Geometry check sheet. Reference: drawing and pictorial views, mm from the part's lowest x, y, z. Coordinates: 2 decimals unless noted, no trailing zeros. Loops run counter-clockwise (first coordinate to the right, second up) from the corner with the lowest first, then second, coordinate; pieces in that order, holes last. Notation, with made-up numbers: (-22, 89) - (1, 89) arc R24 ccw to (1, 100) - close; hole circle Ø7 at (14.25, 34.25). An arc over 180 degrees is marked (long way). One line per item, written item: value.
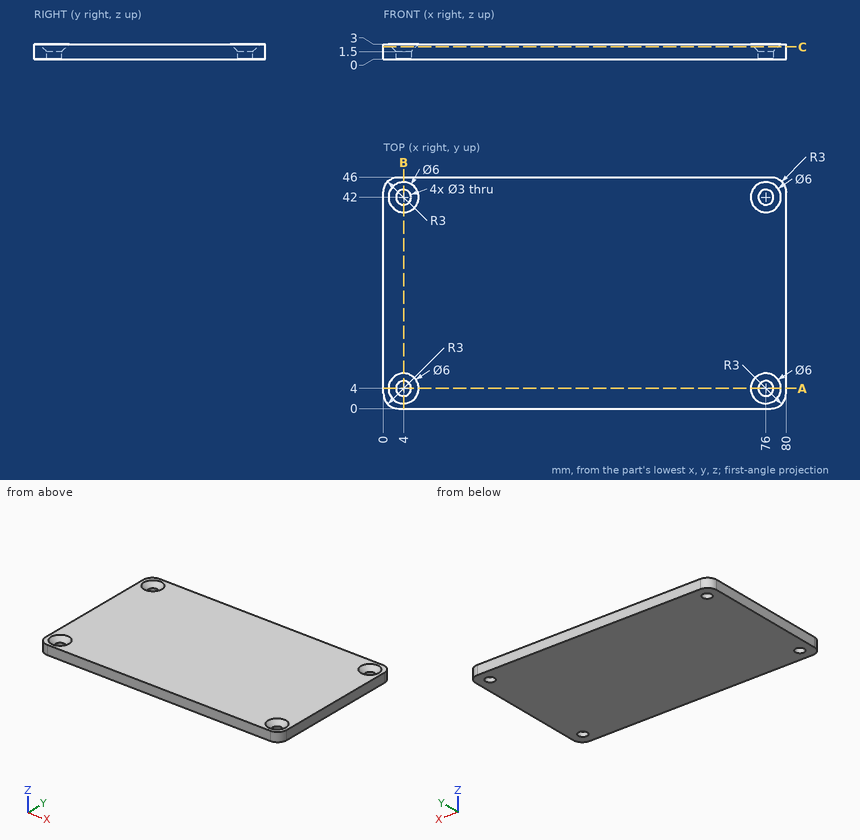
(1) Material ranges on probe 1 along Y at (x, z) = (4, 1.15); probe 2 along Y at (x, z) = (75.5, 2.1); probe 3 along X at (y, z) = (43.5, 2.4), recorded low to high. Write a range as from..to.
Reply:
probe 1: 0..2.5, 5.5..40.5, 43.5..46
probe 2: 0..1.96, 6.04..39.96, 44.04..46
probe 3: 0.04..2.13, 5.87..74.13, 77.87..79.96
(2) Go/stop test with flat-tipped pins: pin 1 Ø2.5 at (x, y) = (4, 42) entering from -Z; pin 2 Ø5 at (x, y) = (4, 4) entering from -Z. Record where each tip stops, or that it passes through.
Reply:
pin 1: through
pin 2: z = 0
(3) Cross-section at B-B on x = 4. Record the cut outline in (y, z).
Reply:
outline: (0, 0) - (2.5, 0) - (2.5, 1.5) - (1, 3) - (0, 3) - close; (5.5, 0) - (40.5, 0) - (40.5, 1.5) - (39, 3) - (7, 3) - (5.5, 1.5) - close; (43.5, 0) - (46, 0) - (46, 3) - (45, 3) - (43.5, 1.5) - close
(4) Cross-section at C-C on z = 2.45. Record the cut outline in (x, y), and give its area (3 significant figures).
Reply:
outline: (0, 3) arc R3 ccw to (3, 0) - (77, 0) arc R3 ccw to (80, 3) - (80, 43) arc R3 ccw to (77, 46) - (3, 46) arc R3 ccw to (0, 43) - close; hole circle Ø4.9 at (4, 4); hole circle Ø4.9 at (4, 42); hole circle Ø4.9 at (76, 4); hole circle Ø4.9 at (76, 42)
area: 3,600 mm2
(5) Cross-section at A-A on y = 4. Record the cut outline in (x, z), and give its area (4 significant figures).
Reply:
outline: (0, 0) - (2.5, 0) - (2.5, 1.5) - (1, 3) - (0, 3) - close; (5.5, 0) - (74.5, 0) - (74.5, 1.5) - (73, 3) - (7, 3) - (5.5, 1.5) - close; (77.5, 0) - (80, 0) - (80, 3) - (79, 3) - (77.5, 1.5) - close
area: 217.5 mm2
